from build123d import *
from build123d.topology import SkipClean

# Parameters (mm, degrees)
SKETCH1_R           = 6.35
BOSS_EXTRUDE1_DEPTH = 25.4
SKETCH3_W           = 3.762901665
SKETCH3_H           = 11.173304621
SKETCH3_W_2         = 4.189249379
CUT_EXTRUDE2_DEPTH  = 25.4
CUT_EXTRUDE3_DEPTH  = 25.4
SKETCH5_R           = 6.35
BOSS_EXTRUDE2_DEPTH = 76.2
FILLET2_R           = 10.16
FILLET3_R           = 10.16
SKETCH6_R           = 4.572
BOSS_EXTRUDE3_DEPTH = 50.8
FILLET5_R           = 10.16


with BuildPart() as part:
    # Sketch1 → Boss-Extrude1 (new body)
    with BuildSketch(Plane(origin=(0, 0, 0), x_dir=(1, 0, 0), z_dir=(0, 1, 0))):
        with Locations(Location((0, 0, 0), (0, 0, 270))):
            Circle(SKETCH1_R)
    extrude(amount=BOSS_EXTRUDE1_DEPTH)

    # Sketch3 → Cut-Extrude2 (cut)
    with BuildSketch(Plane.XZ):
        with Locations((7.723450833, -0.009887881)):
            Rectangle(SKETCH3_W, SKETCH3_H)
        with Locations((-7.93662469, -0.009887881)):
            Rectangle(SKETCH3_W_2, SKETCH3_H)
    extrude(amount=-CUT_EXTRUDE2_DEPTH, mode=Mode.SUBTRACT)

    # Sketch4 → Cut-Extrude3 (cut)
    with BuildSketch(Plane.XZ):
        Polygon((5.523986446, -5.842), (-7.059783038, -5.842), (-7.059783038, -10.872351768), (5.523986446, -11.066959799), align=None)
    cut_extrude3 = extrude(amount=-CUT_EXTRUDE3_DEPTH, mode=Mode.SUBTRACT)

    # Sketch5 → Boss-Extrude2 (add)
    with BuildSketch(Plane(origin=(0, 25.4, 0), x_dir=(1, 0, 0), z_dir=(0, 1, 0))):
        with Locations(Location((0, 0, 0), (0, 0, 66.926081934))):
            Circle(SKETCH5_R)
    extrude(amount=BOSS_EXTRUDE2_DEPTH)

    # Fillet2
    # the kernel refuses this fillet: 10.16 mm, written as the material it adds along each edge
    with BuildSketch(Plane(origin=(-5.842, 25.4, 27.888681579), x_dir=(0, -1, 0), z_dir=(0, 0, -1))) as fillet2_piece_1_section:
        with BuildLine():
            CenterArc((FILLET2_R, FILLET2_R), FILLET2_R, 180, 90)
            Line((0, FILLET2_R), (0, 0))
            Line((0, 0), (FILLET2_R, 0))
        make_face()
    fillet2_piece_1 = extrude(amount=55.777363157, mode=Mode.PRIVATE)
    fillet2_piece_1 = fillet2_piece_1 & Plane(origin=(0, 21.230044771, 0), x_dir=(0, 0, 1), z_dir=(0, -1, 0)) * Cylinder(6.35, 153, mode=Mode.PRIVATE)
    add(fillet2_piece_1)
    with BuildSketch(Plane(origin=(5.842, 25.4, 27.888681579), x_dir=(0, -1, 0), z_dir=(0, 0, -1))) as fillet2_piece_2_section:
        with BuildLine():
            CenterArc((FILLET2_R, -FILLET2_R), FILLET2_R, 90, 90)
            Line((0, -FILLET2_R), (0, 0))
            Line((0, 0), (FILLET2_R, 0))
        make_face()
    fillet2_piece_2 = extrude(amount=55.777363157, mode=Mode.PRIVATE)
    fillet2_piece_2 = fillet2_piece_2 & Plane(origin=(0, 21.230044771, 0), x_dir=(0, 0, 1), z_dir=(0, -1, 0)) * Cylinder(6.35, 153, mode=Mode.PRIVATE)
    add(fillet2_piece_2)

    # Mirror1: Cut-Extrude3 across plane
    with SkipClean():  # the faces are left unmerged after this step: merging them gives an invalid solid
        add(cut_extrude3.mirror(Plane.XY), mode=Mode.SUBTRACT)
    add(part.part.scale(1), mode=Mode.REPLACE)  # the faces are merged on a copy

    # Fillet3
    # the kernel refuses this fillet: 10.16 mm, written as the material it adds along each edge
    with BuildSketch(Plane(origin=(27.888681579, 25.4, 5.842), x_dir=(0, -1, 0), z_dir=(-1, 0, 0))) as fillet3_piece_1_section:
        with BuildLine():
            CenterArc((FILLET3_R, FILLET3_R), FILLET3_R, 180, 90)
            Line((0, FILLET3_R), (0, 0))
            Line((0, 0), (FILLET3_R, 0))
        make_face()
    fillet3_piece_1 = extrude(amount=55.777363157, mode=Mode.PRIVATE)
    fillet3_piece_1 = fillet3_piece_1 & Plane(origin=(0, 21.230043926, 0), x_dir=(0, 0, 1), z_dir=(0, -1, 0)) * Cylinder(6.35, 153, mode=Mode.PRIVATE)
    add(fillet3_piece_1)
    with BuildSketch(Plane(origin=(27.888681579, 25.4, -5.842), x_dir=(0, 0, -1), z_dir=(-1, 0, 0))) as fillet3_piece_2_section:
        with BuildLine():
            CenterArc((FILLET3_R, FILLET3_R), FILLET3_R, 180, 90)
            Line((0, FILLET3_R), (0, 0))
            Line((0, 0), (FILLET3_R, 0))
        make_face()
    fillet3_piece_2 = extrude(amount=55.777363157, mode=Mode.PRIVATE)
    fillet3_piece_2 = fillet3_piece_2 & Plane(origin=(0, 21.230042518, 0), x_dir=(0, 0, 1), z_dir=(0, -1, 0)) * Cylinder(6.35, 153, mode=Mode.PRIVATE)
    add(fillet3_piece_2)

    # Sketch6 → Boss-Extrude3 (add)
    with BuildSketch(Plane(origin=(0, 101.6, 0), x_dir=(1, 0, 0), z_dir=(0, 1, 0))):
        with Locations(Location((0, 0, 0), (0, 0, 270))):
            Circle(SKETCH6_R)
    extrude(amount=BOSS_EXTRUDE3_DEPTH)

    # Fillet5
    # the kernel refuses this fillet: 10.16 mm, written as the material it adds along each edge
    with BuildSketch(Plane(origin=(0, 101.6, 0), x_dir=(0, 0, 1), z_dir=(-1, 0, 0))) as fillet5_piece_1:
        with BuildLine():
            CenterArc((14.732, 5.741748514), FILLET5_R, 180, 34.41150867)
            Line((4.572, 5.741748514), (4.3688, 5.741748514))
            Line((4.3688, 5.741748514), (4.3688, 0))
            Line((4.3688, 0), (4.572, -0.2032))
            ThreePointArc((4.572, -0.2032), (5.461, -0.2032), (6.18236, -0.11483497))
            Line((6.18236, -0.11483497), (6.35, 0))
        make_face()
    revolve(axis=Axis((0, 101.6, 0), (0, 1, 0)))


solid = part.part
Check sheet for the modelled part. Datum: model origin and axes. Units: mm. A direction names the side the tool comes from. Round coordinates to 2 decimals unless told otherwise and drop trailing zeros. Order: outer loops, then holes, each group sorted by start corner. A loop starts at its lowest first (then second) coordinate and runs counter-clockwise, first axis right, second up.
Q1. Depth check by flat-ended pin: P1, Ø5.5, axis at y = 4, z = -0.5, coming from the -X side; P2, Ø2.5, axis at x = 1, y = 6, coming from the -Z side; P3, Ø2, axis at x = 3, y = 49.5, coming from the +Z side. Enter the tip coordinate at first touch or a pass-through.
Filled sheet:
P1: stops at x = -5.84
P2: stops at z = -5.84
P3: stops at z = 6.03
Q2. Scan lines: L1, parallel to Z at x = 2.5, y = 70; L2, parallel to Z at x = 0.5, y = 52. Record each from-to range of solid material in increasing order.
Filled sheet:
L1: z = -5.84 to 5.84
L2: z = -6.33 to 6.33
Q3. Cross-section at C-C, the plane y = 124. Enter the section's corners in (x, z), plus the area to 3 significant figures.
Filled sheet:
outline: circle Ø9.14 at (0, 0)
area: 65.7 mm2
Q4. Cross-section at B-B, the plane x = 0. Enter the section's corners in (y, z).
Filled sheet:
outline: (0, -5.84) - (15.24, -5.84) arc R10.16 cw to (18.41, -6.35) - (101.6, -6.35) arc R10.16 cw to (107.34, -4.57) - (152.4, -4.57) - (152.4, 4.57) - (107.34, 4.57) arc R10.16 cw to (101.6, 6.35) - (18.41, 6.35) arc R10.16 cw to (15.24, 5.84) - (0, 5.84) - close
Q5. Cross-section at A-A, the plane z = 0. Enter the section's corners in (x, y), plus the area to 3 significant figures.
Filled sheet:
outline: (-6.35, 18.41) arc R10.16 cw to (-5.84, 15.24) - (-5.84, 0) - (5.84, 0) - (5.84, 15.24) arc R10.16 cw to (6.35, 18.41) - (6.35, 101.6) arc R10.16 cw to (4.57, 107.34) - (4.57, 152.4) - (-4.57, 152.4) - (-4.57, 107.34) arc R10.16 cw to (-6.35, 101.6) - close
area: 1,740 mm2
Q6. Set-up check for faces 1 (the face through (-5.842, 8, 0)), 2 (the face through (-4.056, 129.555, 2.11)), 3 (the face through (0, 8, -5.842)), 4 (the face through (5.842, 8, 0)), 5 (the face through (0, 8, 5.842)): record each of +Z, -Z, +X, -X, +Y, -Y from which the full face is reachable in a straight line by a thin tool's end or side.
Filled sheet:
face 1: +Z, -Z, -X, -Y
face 2: +Y
face 3: -Z, +X, -X, -Y
face 4: +Z, -Z, +X, -Y
face 5: +Z, +X, -X, -Y
Q7. Cross-section at D-D, the plane y = 46. Enter the section's corners in (x, z), plus the area to 3 significant figures.
Filled sheet:
outline: circle Ø12.7 at (0, 0)
area: 127 mm2
